Model file for the job. Use its own axes, mm. A direction names the side the tool comes from. Round coordinates to 2 decimals unless told otherwise and drop trailing zeros. Order: outer loops, then holes, each group sorted by start corner. A loop starts at its lowest first (then second) coordinate and runs counter-clockwise, first axis right, second up. Notation, with made-up numbers: (50.25, 78) - (107.25, 78) arc R18 cw to (107.25, 90) - close; hole circle Ø3 at (43.25, 74). An arc over 180 degrees is marked (long way). Put each result on its own line as item: value. Start each with the question number.
Item 1: Saw through at B-B on z = 2.2. List the corners of the cut face in (x, y), plus the area to 3 significant figures.
Item 2: Saw through at A-A on y = 46. List the corners of the cut face in (x, z), plus the area to 3 significant figures.
Item 3: Probe probe 1 along X at (y, z) = (37, 1); probe 2 along X at (y, z) = (13, 3.8); probe 3 along Y at (x, z) = (13.5, 2.7). List the from-to ranges inside material, lowest first.
Item 4: Mould opens along Y. For faces 4 (the face through (21, 50.556, 2)), 5 (the face through (14.1, 19.89, 3.02)), 6 (the face through (14.05, 18.83, 1.78)) say: pulls with the +Y half, pulls with the -Y half, needs draft (parallel to the pull), parting line crosses it, or undercut.
Item 5: Pin check, flat tips, straight feed: pin 1 Ø2.5 at (y, z) = (40.5, 2.5) entering from -X; pin 2 Ø2.5 at (y, z) = (49, 2) entering from -X; pin 3 Ø2.5 at (y, z) = (13.5, 2.5) entering from -X. Stop position of each tip, or through.
Item 6: Saw through at C-C on x = 64.5. List the corners of the cut face in (y, z).
Item 7: Saw through at D-D on x = 35.5. List the corners of the cut face in (y, z).
Item 8: Which spindle directions (+Z, -Z, +X, -X, +Y, -Y) get a long thin tool onto all of the face, cutting with end or side? Do faces 1 (the face through (25.556, 30, 2)), 2 (the face through (14.05, 48.83, 1.78)), 3 (the face through (15.556, 34, 2)). Say none if no direction does.
```python
from build123d import *

# Parameters (mm, degrees)
F0_R     = 3.350006
F1_DEPTH = 5
F3_DEPTH = 40.5559613398
F5_DEPTH = 15.5559613398


# Not quite as in the source:
# - a feature names something its author has since deleted; it is built from what else it names


with BuildPart() as f1:
    # F0 (on Top) → F1 (new body)
    with BuildSketch(Plane.XY):
        Polygon((0, 10), (3.4919226796, 10), (1.7459613398, 13.81), align=None)
        Polygon((15.5559613398, 18.81), (15.5559613398, 20.5559613398), (11.7459613398, 18.81), align=None)
        Polygon((15.5559613398, 47.0640386602), (15.5559613398, 50.5559613398), (11.7459613398, 48.81), align=None)
        Polygon((25.5559613398, 50.5559613398), (15.5559613398, 50.5559613398), (15.5559613398, 47.0640386602), (15.5559613398, 20.5559613398), (15.5559613398, 18.81), (15.5559613398, 17.0640386602), (15.5559613398, 10), (3.4919226796, 10), (0, 10), (0, 0), (76.6976781032, 0), (76.6976781032, 67.5584669805), (56.6976781032, 67.5584669805), (56.6976781032, 10), (25.5559613398, 10), align=None)
        with Locations((66.6976781032, 8.7792334903)):
            Circle(F0_R, mode=Mode.SUBTRACT)
        with Locations((66.6976781032, 58.7792334903)):
            Circle(F0_R, mode=Mode.SUBTRACT)
        Polygon((15.5559613398, 17.0640386602), (15.5559613398, 18.81), (11.7459613398, 18.81), align=None)
    extrude(amount=F1_DEPTH)

    # F2 (on face) → F3 (cut, through all)
    with BuildSketch(Plane(origin=(0, 50.5559613398, 0), x_dir=(-1, 0, 0), z_dir=(0, 1, 0))):
        Polygon((-11.7459613398, 4.5), (-15.5559613398, 0), (-11.7459613398, 0), align=None)
    extrude(amount=-F3_DEPTH, mode=Mode.SUBTRACT)

    # F4 (on face) → F5 (cut, through all)
    with BuildSketch(Plane(origin=(0, 0, 0), x_dir=(0, -1, 0), z_dir=(-1, 0, 0))):
        Polygon((-13.81, 0), (-10, 0), (-13.81, 4.5), align=None)
    extrude(amount=-F5_DEPTH, mode=Mode.SUBTRACT)


solid = f1.part
```
Results found:
1. outline: (0, 0) - (76.7, 0) - (76.7, 67.56) - (56.7, 67.56) - (56.7, 10) - (25.56, 10) - (25.56, 50.56) - (15.56, 50.56) - (13.69, 49.7) - (13.69, 47.92) - (15.56, 47.06) - (15.56, 20.56) - (13.69, 19.7) - (13.69, 17.92) - (15.56, 17.06) - (15.56, 10) - (3.49, 10) - (2.64, 11.86) - (0.85, 11.86) - (0, 10) - close; hole circle Ø6.7 at (66.7, 8.78); hole circle Ø6.7 at (66.7, 58.78)
1. area: 2,270 mm²
2. outline: (15.56, 0) - (25.56, 0) - (25.56, 5) - (15.56, 5) - close; (56.7, 0) - (76.7, 0) - (76.7, 5) - (56.7, 5) - close
2. area: 150 mm²
3. probe 1: x = 15.56 to 25.56, 56.7 to 76.7
3. probe 2: x = 1.37 to 2.12, 15.56 to 25.56, 56.7 to 76.7
3. probe 3: y = 0 to 10, 18.01 to 19.61, 48.01 to 49.61
4. face 4: pulls with the +Y half
4. face 5: undercut
4. face 6: needs draft
5. pin 1: stops at x = 15.56
5. pin 2: stops at x = 12.8
5. pin 3: stops at x = 1.04
6. outline: (0, 0) - (6.25, 0) - (6.25, 5) - (0, 5) - close; (11.31, 0) - (56.25, 0) - (56.25, 5) - (11.31, 5) - close; (61.31, 0) - (67.56, 0) - (67.56, 5) - (61.31, 5) - close
7. outline: (0, 0) - (10, 0) - (10, 5) - (0, 5) - close
8. face 1: +Z, -Z, +Y
8. face 2: -Z, -X, +Y
8. face 3: +Z, -Z, -X
